CAD build for the part. Positions are in the model's coordinates, mm. A direction names the side the tool comes from. Round coordinates to 2 decimals unless told otherwise and drop trailing zeros. Order: outer loops, then holes, each group sorted by start corner. A loop starts at its lowest first (then second) coordinate and runs counter-clockwise, first axis right, second up. Notation, with made-up numbers: M -17.5,-2 L -13.5,-2 A18 ccw -13.5,27 Z; hole C 74.25,58.5 d5. An arc over 180 degrees is marked long. Answer as CSV lines item,"result". Start each with the question number.
```python
from build123d import *

# Parameters (mm, degrees)
SKETCH2_R            = 4.5
BOSS_EXTRUDE1_DEPTH  = 15
SKETCH6_W            = 18
SKETCH6_H            = 16
SKETCH6_H_2          = 3
BOSS_EXTRUDE9_DEPTH  = 33
CUT_EXTRUDE2_DEPTH   = 33
BOSS_EXTRUDE11_DEPTH = 15
BOSS_EXTRUDE13_DEPTH = 24
SKETCH20_W           = 24
SKETCH20_H           = 12
CUT_EXTRUDE3_DEPTH   = 57
BOSS_EXTRUDE15_DEPTH = 15
SKETCH22_R           = 3
CUT_EXTRUDE4_DEPTH   = 47


with BuildPart() as part:
    # Sketch2 → Boss-Extrude1 (new body)
    with BuildSketch(Plane.XY):
        with BuildLine():
            Line((-78.062958061, 34.644624266), (-78.062958061, 25.644624266))
            Line((-78.062958061, 25.644624266), (-60.062958061, 25.644624266))
            Line((-60.062958061, 25.644624266), (-60.062958061, 34.644624266))
            ThreePointArc((-60.062958061, 34.644624266), (-69.062958061, 43.644624266), (-78.062958061, 34.644624266))
        make_face()
        with Locations((-69.062958061, 34.644624266)):
            Circle(SKETCH2_R, mode=Mode.SUBTRACT)
    extrude(amount=-BOSS_EXTRUDE1_DEPTH)

    # Sketch6 → Boss-Extrude9 (add)
    with BuildSketch(Plane(origin=(0, 0, -15), x_dir=(-1, 0, 0), z_dir=(0, 0, -1))):
        with Locations((69.062958061, 14.644624266)):
            Rectangle(SKETCH6_W, SKETCH6_H)
        with Locations((69.062958061, 24.144624266)):
            Rectangle(SKETCH6_W, SKETCH6_H_2)
    extrude(amount=-BOSS_EXTRUDE9_DEPTH)

    # Sketch15 → Cut-Extrude2 (cut)
    with BuildSketch(Plane.ZY.offset(78.062958061)):
        Polygon((-15, 6.644624266), (-15, 22.644624266), (3, 6.644624266), align=None)
        Polygon((18, 9.644624266), (0, 25.644624266), (18, 25.644624266), align=None)
    extrude(amount=-CUT_EXTRUDE2_DEPTH, mode=Mode.SUBTRACT)

    # Sketch16 → Boss-Extrude11 (add)
    with BuildSketch(Plane.XY.offset(18)):
        with BuildLine():
            Line((-78.062958061, 6.644624266), (-78.062958061, 0.644624266))
            ThreePointArc((-78.062958061, 0.644624266), (-74.548239436, -7.840657108), (-66.062958061, -11.355375734))
            Line((-66.062958061, -11.355375734), (-7.062958061, -11.355375734))
            Line((-7.062958061, -11.355375734), (-7.062958061, 6.644624266))
            Line((-7.062958061, 6.644624266), (-78.062958061, 6.644624266))
        make_face()
    extrude(amount=-BOSS_EXTRUDE11_DEPTH)

    # Sketch18 → Boss-Extrude13 (add)
    with BuildSketch(Plane.XY.offset(18)):
        Polygon((28.937041939, -11.355375734), (-7.062958061, -11.355375734), (-7.062958061, 6.644624266), (-7.062958061, 28.644624266), (28.937041939, 28.644624266), align=None)
    extrude(amount=-BOSS_EXTRUDE13_DEPTH)

    # Sketch20 → Cut-Extrude3 (cut)
    with BuildSketch(Plane(origin=(0, 28.644624266, 0), x_dir=(1, 0, 0), z_dir=(0, 1, 0))):
        with Locations((10.937041939, -6)):
            Rectangle(SKETCH20_W, SKETCH20_H)
    extrude(amount=-CUT_EXTRUDE3_DEPTH, mode=Mode.SUBTRACT)

    # Sketch21 → Boss-Extrude15 (add)
    with BuildSketch(Plane.XY):
        with BuildLine():
            Line((22.937041939, 28.644624266), (34.937041939, 28.644624266))
            Line((34.937041939, 28.644624266), (34.937041939, 64.644624266))
            Line((34.937041939, 64.644624266), (48.937041939, 64.644624266))
            Line((48.937041939, 64.644624266), (48.937041939, 49.588896176))
            ThreePointArc((48.937041939, 49.588896176), (49.937041939, 31.644624266), (50.937041939, 49.588896176))
            Line((50.937041939, 49.588896176), (50.937041939, 64.644624266))
            Line((50.937041939, 64.644624266), (64.937041939, 64.644624266))
            Line((64.937041939, 64.644624266), (64.937041939, 20.644624266))
            ThreePointArc((64.937041939, 20.644624266), (55.564458937, -1.982792732), (32.937041939, -11.355375734))
            Line((32.937041939, -11.355375734), (22.937041939, -11.355375734))
            Line((22.937041939, -11.355375734), (22.937041939, 28.644624266))
        make_face()
    extrude(amount=BOSS_EXTRUDE15_DEPTH)

    # Sketch22 → Cut-Extrude4 (cut)
    with BuildSketch(Plane(origin=(64.937041939, 0, 0), x_dir=(0, 0, -1), z_dir=(1, 0, 0))):
        with Locations((-7.5, 58.644624266)):
            Circle(SKETCH22_R)
    extrude(amount=-CUT_EXTRUDE4_DEPTH, mode=Mode.SUBTRACT)


solid = part.part
```
Q1. Mould opens along X. For faces 1 (the flat face through (-60.063, 21, -2)), 2 (the flat face through (-16, -11.355, 9)), 3 (the flat face through (34.937, 46, 7)) say: +X half, -X half, draft (parallel to the pull), parting line (faces both ways), or undercut.
Q2. Band-saw the part on C-C, the plane y = 24. Write the cut outline in (x, z).
Q3. Drop flat-ended pins along their axis: P1, Ø5, axis at y = 3.5, z = -5.5, coming from the -X side; P2, Ø1, axis at x = -60, y = 30, coming from the +Z side; P3, Ø3.5, axis at y = 17.5, z = 4.5, coming from the +X side; P4, Ø6, axis at y = 2.5, z = 0.5, coming from the -X side. Give the stop position or say it passes through.
Q4. Band-saw the part on B-B, the plane x = 44.5. Write the cut outline in (y, z), then the cut area to 3 significant figures.
Q5. Band-saw the part on D-D, the plane z = -12.5. Write the cut outline in (x, y), then the cut area to 3 significant figures.
Q6. Tool access for faces 4 (the flat face through (47, 27, 0)), 5 (the flat face through (-7.063, 13, 4)), 6 (the flat face through (48.937, 55.5, 5.7)), 7 (the flat face through (-43, -2, 3)), 8 (the flat face through (11, 9, 0)): list every direction of +Z, -Z, +X, -X, +Y, -Y with a clear straight run to the whole face (end or side of a thin tool).
Q7. Probe line 1 along Z through (x, y) = (12, -0.5); line 2 along Y through (x, z) = (43.5, 7.5); line 3 along X through (y, z) = (56.5, 5). List the from-to ranges inside material, lowest first. Write a range as from..to.
Q8. Band-saw the part on A-A, the plane y = 54. Write the cut outline in (x, z).
Answer:
1,face 1,"undercut"
1,face 2,"draft"
1,face 3,"-X half"
2,outline,"M -78.06,-15 L -60.06,-15 L -60.06,1.85 L -78.06,1.85 Z; M -7.06,-6 L 28.94,-6 L 28.94,0 L 64.94,0 L 64.94,15 L 28.94,15 L 28.94,18 L -7.06,18 Z; hole M -1.06,0 L 22.94,0 L 22.94,12 L -1.06,12 Z"
3,P1,"stops at x = -7.06"
3,P2,"stops at z = 0"
3,P3,"stops at x = 64.91"
3,P4,"stops at x = -78.06"
4,outline,"M -9.19,0 L 33.47,0 L 33.47,15 L -9.19,15 Z; M 47.82,0 L 64.64,0 L 64.64,15 L 47.82,15 Z; hole C 58.64,7.5 d6"
4,area,"864 mm^2"
5,outline,"M -78.06,20.42 L -60.06,20.42 L -60.06,34.64 A9 ccw -78.06,34.64 Z; hole C -69.06,34.64 d9"
5,area,"320 mm^2"
6,face 4,"-Z, +X, +Y, -Y"
6,face 5,"-Z, +Y"
6,face 6,"+Z, -Z, +Y"
6,face 7,"-Z, -X, -Y"
6,face 8,"+Y, -Y"
7,line 1,"z = -6..0, 12..18"
7,line 2,"y = -9.56..34.35, 46.93..55.64, 61.64..64.64"
7,line 3,"x = 34.94..48.94, 50.94..64.94"
8,outline,"M 34.94,0 L 48.94,0 L 48.94,15 L 34.94,15 Z; M 50.94,0 L 64.94,0 L 64.94,15 L 50.94,15 Z"
